from build123d import *

# Parameters (mm, degrees)
SKETCH_3_R      = 40
EXTRUDE_1_DEPTH = 20
SKETCH_4_W      = 80
SKETCH_4_H      = 20
EXTRUDE_2_DEPTH = 80
FILLET_2_R      = 10
FILLET_3_R      = 30


with BuildPart() as part:
    # 草图3 → 凸台-拉伸1 (new body)
    with BuildSketch(Plane(origin=(0, 0, 0), x_dir=(1, 0, 0), z_dir=(0, 1, 0))):
        with BuildLine():
            Line((-40, 71.189389762), (-40, 0))
            ThreePointArc((-40, 0), (0, 40), (40, 0))
            Line((40, 0), (40, 71.189389762))
            Line((40, 71.189389762), (-40, 71.189389762))
        make_face()
        Circle(SKETCH_3_R)
    extrude(amount=EXTRUDE_1_DEPTH)

    # 草图4 → 凸台-拉伸2 (add)
    with BuildSketch(Plane(origin=(0, 20, 0), x_dir=(1, 0, 0), z_dir=(0, 1, 0))):
        with Locations((0, 61.189389762)):
            Rectangle(SKETCH_4_W, SKETCH_4_H)
    extrude(amount=EXTRUDE_2_DEPTH)

    # 圆角2
    fillet_2_edges = [part.edges().sort_by_distance(p)[0] for p in [
        (0, 20, -51.189389762),
    ]]
    fillet(fillet_2_edges, radius=FILLET_2_R)

    # 圆角3
    fillet_3_edges = [part.edges().sort_by_distance(p)[0] for p in [
        (0, 0, -71.189389762),
    ]]
    fillet(fillet_3_edges, radius=FILLET_3_R)


solid = part.part
Geometry: final body of the model. Coordinates: model frame, mm. A direction names the side the tool comes from. Round coordinates to 2 decimals unless told otherwise and drop trailing zeros. Order: outer loops, then holes, each group sorted by start corner. A loop starts at its lowest first (then second) coordinate and runs counter-clockwise, first axis right, second up.
Q1. Pin query (flat end, axial travel): pin 1 (5 mm diameter, centred on x = -14.5, y = 17.5, fed in from +Z); pin 2 (2 mm diameter, centred on x = 19.5, y = 22, fed in from +Z); pin 3 (6 mm diameter, centred on x = -24, y = 76.5, fed in from +Z). Return the tip coordinate at first contact, or that it passes through.
Result sheet:
pin 1: stops at z = 38.16
pin 2: stops at z = -45.55
pin 3: stops at z = -51.19
Q2. Access query for faces 1 (the face through (-1, 20, -1)), 2 (the face through (40, 27, -51)). Directions: +Z, -Z, +X, -X, +Y, -Y. A direction counts if a zero-diameter tool reaches every point of the face in a straight line with its end or side. Return the directions, or none.
Result sheet:
face 1: +Z, +X, -X, +Y
face 2: +Z, -Z, +X, +Y, -Y
Q3. Section A-A, the plane x = 0. Output: boundary loops of the cut face in (y, z), and give its area (3 significant figures).
Result sheet:
outline: (0, -41.19) arc R30 ccw to (30, -71.19) - (100, -71.19) - (100, -51.19) - (30, -51.19) arc R10 cw to (20, -41.19) - (20, 40) - (0, 40) - close
area: 3,650 mm2
Q4. Section B-B, the plane y = 48.5. Output: boundary loops of the cut face in (x, z), and give its area (3 significant figures).
Result sheet:
outline: (-40, -71.19) - (40, -71.19) - (40, -51.19) - (-40, -51.19) - close
area: 1,600 mm2
Q5. Section D-D, the plane x = -12. Output: boundary loops of the cut face in (y, z).
Result sheet:
outline: (0, -41.19) arc R30 ccw to (30, -71.19) - (100, -71.19) - (100, -51.19) - (30, -51.19) arc R10 cw to (20, -41.19) - (20, 38.16) - (0, 38.16) - close
Q6. Section C-C, the plane z = -15. Output: boundary loops of the cut face in (x, y).
Result sheet:
outline: (-40, 0) - (40, 0) - (40, 20) - (-40, 20) - close
Q7. Material intervals for probe 1 along Z at (x, y) = (-25, 68.5); probe 2 along Y at (x, z) = (-10.5, 27.5); probe 3 along Z at (x, y) = (18, 9), sorted ascending.
Result sheet:
probe 1: z = -71.19 to -51.19
probe 2: y = 0 to 20
probe 3: z = -62.61 to 35.72
